Can you work these out from the model? Positions are in its coordinate system, mm. Round coordinates to 2 decimals unless told otherwise and drop trailing zeros. Order: outer loops, then holes, each group sorted by start corner. A loop starts at its lowest first (then second) coordinate and runs counter-clockwise, first axis right, second up. Notation, with made-up numbers: (11, 81) -> (33, 81) arc R28 ccw to (33, 110) -> close; hole circle Ø10 at (6.25, 13). An arc over 180 degrees is marked (long way). One line per item, written item: value.
Autodesk Inventor part; units mm, degrees
ref_plane "Work Plane1" through (0, 50.8, 0) normal (0, 1, 0) x (-1, 0, 0)
ref_plane "YZ Plane" through (0, 0, 0) normal (1, 0, 0) x (0, 1, 0)
ref_plane "XY Plane" through (0, 0, 0) normal (0, 0, 1) x (1, 0, 0)
sketch "Sketch1" plane through (0, 0, 0) normal (0, 0, 1) x (1, 0, 0)
  circle A0 centre (0, 0) radius 50.8
  circle A1 centre (0, 0) radius 47.625
  dimension "d0" = 101.6
  dimension "d1" = 95.25
extrude "Extrusion1" add sketch "Sketch1" along normal blind 711.2
ref_plane "Work Plane1" through (0, 50.8, 0) normal (0, 1, 0) x (-1, 0, 0)
sketch "Sketch5" plane through (0, 0, 0) normal (1, 0, 0) x (0, 1, 0)
  line L0 (50.8, 711.2) -> (-50.8, 711.2) construction
  line L1 (-50.8, 0) -> (50.8, 0) construction
  line L2 (3.175, 711.2) -> (-3.175, 711.2)
  line L3 (-3.175, 711.2) -> (-3.175, 679.45)
  line L4 (3.175, 679.45) -> (3.175, 711.2)
  arc A0 (-3.175, 679.45) -> (3.175, 679.45) centre (0, 679.45) ccw
  line L5 (0, 769.9295) -> (0, 0) construction
  dimension "d16" = 3.175
  dimension "d17" = 31.75
extrude "Extrusion4" cut sketch "Sketch5" along normal through all both and the other way through all
sketch "Sketch6" plane through (0, 0, 0) normal (0, 1, 0) x (-1, 0, 0)
  line L0 (4.7625, 203.2) -> (4.7625, 165.1)
  line L1 (-4.7625, 203.2) -> (-4.7625, 165.1)
  arc A0 (4.7625, 203.2) -> (-4.7625, 203.2) centre (0, 203.2) ccw
  arc A1 (-4.7625, 165.1) -> (4.7625, 165.1) centre (0, 165.1) ccw
  point P0 (0, 0)
  dimension "d20" = 203.2
  dimension "d21" = 165.1
  dimension "d22" = 9.525
extrude "Extrusion5" cut sketch "Sketch6" against normal through all
sketch "Sketch7" plane through (0, 50.8, 0) normal (0, 1, 0) x (-1, 0, 0)
  line L0 (4.7625, 161.925) -> (4.7625, 107.95)
  line L1 (-4.7625, 107.95) -> (-4.7625, 161.925)
  arc A0 (-4.7625, 107.95) -> (4.7625, 107.95) centre (0, 107.95) ccw
  arc A1 (4.7625, 161.925) -> (-4.7625, 161.925) centre (0, 161.925) ccw
  line L2 (-50.8, 0) -> (50.8, 0)
  point P0 (0, 0)
  dimension "d25" = 107.95
  dimension "d26" = 161.925
  dimension "d27" = 9.525
extrude "Extrusion6" cut sketch "Sketch7" against normal blind 25.4
properties part number "PrimaryHullLexanTube_01" material "Polycarbonate, Clear"
Q1. I want a section at B-B on z = 262.5. List the corners of the cut face in (x, y) for me (3 decimals).
Answers below:
outline: circle Ø101.6 at (0, 0); hole circle Ø95.25 at (0, 0)
Q2. Will these pins go through, and if not, where does the flat tip stop? pin 1 Ø5 at (x, z) = (-13.5, 310) entering from -Y; pin 2 Ø8 at (x, z) = (32.5, 91.5) entering from +Y; pin 3 Ø1.5 at (y, z) = (-17.5, 130.5) entering from +X; pin 4 Ø4 at (x, y) = (40.5, -20.5) entering from -Z.
Answers below:
pin 1: y = -49.59
pin 2: y = 42.05
pin 3: x = 47.96
pin 4: through
Q3. I want a section at A-A on x = 22. List the corners of the cut face in (y, z) for me, plus the area to 3 significant figures.
Answers below:
outline: (-45.79, 0) -> (-42.24, 0) -> (-42.24, 711.2) -> (-45.79, 711.2) -> close; (42.24, 0) -> (45.79, 0) -> (45.79, 711.2) -> (42.24, 711.2) -> close
area: 5,050 mm^2
Q4. Please list where these lines run through material, in increasing order: line 1 along X through (y, z) = (5, 226.5); line 2 along Y through (x, z) = (0, 387.5) (3 decimals).
Answers below:
line 1: -50.55 to -47.36, 47.36 to 50.55
line 2: -50.8 to -47.625, 47.625 to 50.8
Q5. We'd pull the mould along X, two halves only. Please class faces 1 (the face through (-15.3, 45.4, 0)), 2 (the face through (-11.012, 49.592, 350.622)), 3 (the face through (-37.794, 28.979, 350.622)): released by +X, released by -X, zero draft, split by the parting line, or undercut.
Answers below:
face 1: zero draft
face 2: split by the parting line
face 3: undercut
Q6. I want a section at D-D on x = -31.5. List the corners of the cut face in (y, z) for me.
Answers below:
outline: (-39.85, 0) -> (-35.72, 0) -> (-35.72, 711.2) -> (-39.85, 711.2) -> close; (35.72, 0) -> (39.85, 0) -> (39.85, 711.2) -> (35.72, 711.2) -> close
